Print and shaded views of the part. All mm, measured from the part's lowest x, y and z. Coordinates: 2 decimals unless noted, no trailing zeros. Order: outer loops, then holes, each group sorted by start corner. A loop starts at its lowest first (then second) coordinate and runs counter-clockwise, first axis right, second up.
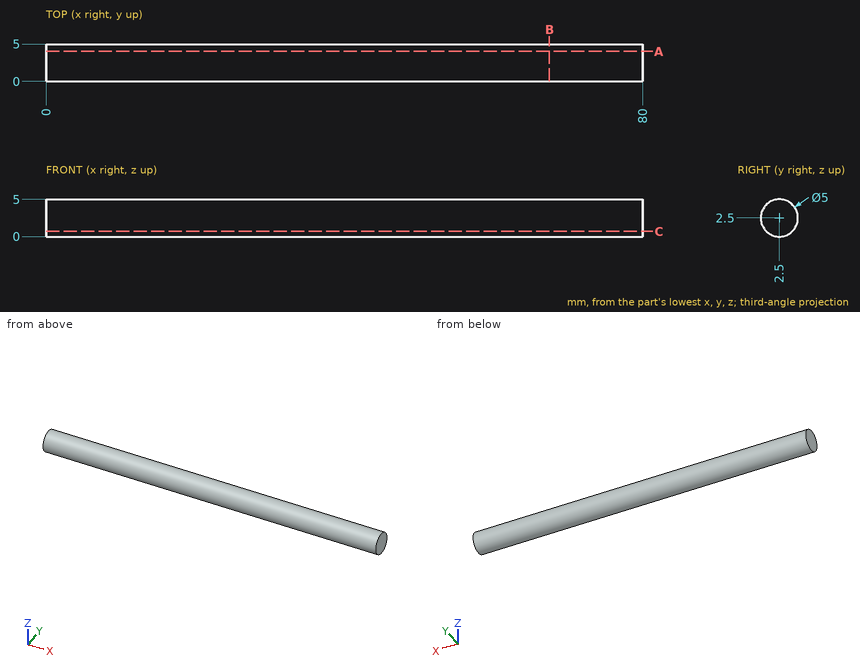
Q1. Cut at C-C, the plane z = 0.7. List the corners of the cut face in (x, y).
Established:
outline: (0, 0.77) - (80, 0.77) - (80, 4.23) - (0, 4.23) - close
Q2. Cut at B-B, the plane x = 67.5. List the corners of the cut face in (y, z).
Established:
outline: circle Ø5 at (2.5, 2.5)
Q3. Probe line 1 (Z direction, x = 63.5, y = 2.35); line 2 (Y direction, x = 67, z = 2.75); line 3 (Z direction, x = 76.5, y = 3.4). List the from-to ranges inside material, lowest first.
Established:
line 1: z = 0 to 5
line 2: y = 0.01 to 4.99
line 3: z = 0.17 to 4.83
Q4. Drop flat-ended pins along their axis: P1, Ø2, axis at y = 3.5, z = 1, coming from the -X side; P2, Ø2, axis at x = 69.5, y = 4, coming from the -Z side. Give the stop position or say it passes through.
Established:
P1: stops at x = 0
P2: stops at z = 0.05
Q5. Cut at A-A, the plane y = 4. List the corners of the cut face in (x, z), plus the area to 3 significant figures.
Established:
outline: (0, 0.5) - (80, 0.5) - (80, 4.5) - (0, 4.5) - close
area: 320 mm2
